Design review of the part built by this model. Coordinates are the model's own, in mm. Give positions to 0.01 mm unless a question says otherwise; leave off trailing zeros. Order: outer loops, then holes, each group sorted by start corner. A loop starts at its lowest first (then second) coordinate and runs counter-clockwise, first axis right, second up. Notation, with made-up numbers: (89.5, -11) -> (100.5, -11) arc R15 ccw to (100.5, 12) -> close; hole circle Ø9 at (88, -19.75). An arc over 180 degrees is marked (long way). One line per item, written item: value.
from build123d import *

# Parameters (mm, degrees)
SZKIC1_R                        = 6
SZKIC1_R_2                      = 1.6
SZKIC1_R_3                      = 2.15
DODANIE_WYCI_GNI_CIE1_DEPTH     = 5
ZAOKR_GLENIE1_R                 = 20
SFAZOWANIE1_SIZE                = 1
SZKIC2_R                        = 3.05
WYTNIJ_WYCI_GNI_CIE1_DEPTH      = 1.0000001
WYTNIJ_WYCI_GNI_CIE1_DEPTH_BACK = 6.0000001
SZKIC3_R                        = 2.25
WYTNIJ_WYCI_GNI_CIE2_DEPTH      = 1.0000001
WYTNIJ_WYCI_GNI_CIE2_DEPTH_BACK = 6.0000001
SZKIC4_R                        = 5
WYTNIJ_WYCI_GNI_CIE3_DEPTH      = 16
SZKIC5_R                        = 6
WYTNIJ_WYCI_GNI_CIE4_DEPTH      = 10
SZKIC6_R                        = 1.575
WYTNIJ_WYCI_GNI_CIE5_DEPTH      = 10
SFAZOWANIE2_SIZE                = 1


with BuildPart() as part:
    # Szkic1 → Dodanie-wyci_gni_cie1 (new body)
    with BuildSketch(Plane.XY):
        with BuildLine():
            ThreePointArc((117.467013895, 64.47868366), (93.021164267, 71.454105589), (67.678172045, 73.451308732))
            Line((67.678172045, 73.451308732), (-67.678172045, 73.451308732))
            ThreePointArc((-67.678172045, 73.451308732), (-93.021164267, 71.454105589), (-117.467013895, 64.47868366))
            ThreePointArc((-117.467013895, 64.47868366), (-133.996600631, 0.95447329), (-118.373625878, -62.798763495))
            ThreePointArc((-118.373625878, -62.798763495), (-114.037971639, -67.832241049), (-107.953613934, -70.499521549))
            ThreePointArc((-107.953613934, -70.499521549), (0, -80.778253493), (107.953613934, -70.499521549))
            ThreePointArc((107.953613934, -70.499521549), (114.037971639, -67.832241049), (118.373625878, -62.798763495))
            ThreePointArc((118.373625878, -62.798763495), (133.996600631, 0.95447329), (117.467013895, 64.47868366))
        make_face()
        with Locations((-79.843156229, -62.51471301)):
            Circle(SZKIC1_R, mode=Mode.SUBTRACT)
        with Locations((-60, -65.014543178)):
            Circle(SZKIC1_R, mode=Mode.SUBTRACT)
        with BuildLine():
            Line((-93.639920436, -10.215979742), (-85.426816489, -11.936656557))
            ThreePointArc((-85.426816489, -11.936656557), (-69.154538898, -19.133220925), (-57.227836692, -32.336679986))
            add(Edge.make_bspline(
                [(-72.285057891, -50.981377576), (-64.366611345, -52.03697099), (-50.388689008, -44.15086566), (-57.227836692, -32.336679986)],
                knots=[0, 0, 0, 0, 1, 1, 1, 1], degree=3))
            ThreePointArc((-72.285057891, -50.981377576), (-83.943779984, -49.299228552), (-95.563579221, -47.366434753))
            ThreePointArc((-95.563579221, -47.366434753), (-101.119264644, -44.79470717), (-104.683334782, -39.817074466))
            ThreePointArc((-104.683334782, -39.817074466), (-107.042286981, -32.953737236), (-108.951787413, -25.952033051))
            ThreePointArc((-108.951787413, -25.952033051), (-105.622705702, -13.873790687), (-93.639920436, -10.215979742))
        make_face(mode=Mode.SUBTRACT)
        with Locations((60, -65.014543178)):
            Circle(SZKIC1_R, mode=Mode.SUBTRACT)
        with Locations((79.843156229, -62.51471301)):
            Circle(SZKIC1_R, mode=Mode.SUBTRACT)
        with BuildLine():
            ThreePointArc((57.227836692, -32.336679986), (69.154538898, -19.133220925), (85.426816489, -11.936656557))
            Line((85.426816489, -11.936656557), (93.639920436, -10.215979742))
            ThreePointArc((93.639920436, -10.215979742), (105.622705702, -13.873790687), (108.951787413, -25.952033051))
            ThreePointArc((108.951787413, -25.952033051), (107.042286981, -32.953737236), (104.683334782, -39.817074466))
            ThreePointArc((104.683334782, -39.817074466), (101.119264644, -44.79470717), (95.563579221, -47.366434753))
            ThreePointArc((95.563579221, -47.366434753), (83.943779984, -49.299228552), (72.285057891, -50.981377576))
            add(Edge.make_bspline(
                [(72.285057891, -50.981377576), (64.366611345, -52.03697099), (50.388689008, -44.15086566), (57.227836692, -32.336679986)],
                knots=[0, 0, 0, 0, 1, 1, 1, 1], degree=3))
        make_face(mode=Mode.SUBTRACT)
        with BuildLine():
            Line((-74.826032056, 11.014530402), (-96.655711946, 16.415211274))
            ThreePointArc((-96.655711946, 16.415211274), (-105.521825108, 23.188783802), (-106.621107385, 34.291973698))
            ThreePointArc((-106.621107385, 34.291973698), (-104.340687454, 40.706522101), (-101.674756414, 46.970670723))
            ThreePointArc((-101.674756414, 46.970670723), (-91.74794023, 55.218917354), (-79.089039168, 52.703469899))
            ThreePointArc((-79.089039168, 52.703469899), (-75.870232147, 50.506568408), (-72.478506287, 48.587378348))
            ThreePointArc((-72.478506287, 48.587378348), (-63.066485572, 41.379596603), (-56.80899086, 31.310733134))
            add(Edge.make_bspline(
                [(-58.521368144, 15.244283258), (-55.163116948, 18.373947188), (-54.683502949, 25.918210288), (-56.80899086, 31.310733134)],
                knots=[0, 0, 0, 0, 1, 1, 1, 1], degree=3))
            ThreePointArc((-58.521368144, 15.244283258), (-66.137786774, 11.063591883), (-74.826032056, 11.014530402))
        make_face(mode=Mode.SUBTRACT)
        with BuildLine():
            Line((96.655711946, 16.415211274), (74.826032056, 11.014530402))
            ThreePointArc((74.826032056, 11.014530402), (66.137786774, 11.063591883), (58.521368144, 15.244283258))
            add(Edge.make_bspline(
                [(58.521368144, 15.244283258), (55.163116948, 18.373947188), (54.683502949, 25.918210288), (56.80899086, 31.310733134)],
                knots=[0, 0, 0, 0, 1, 1, 1, 1], degree=3))
            ThreePointArc((56.80899086, 31.310733134), (63.066485572, 41.379596603), (72.478506287, 48.587378348))
            ThreePointArc((72.478506287, 48.587378348), (75.870232147, 50.506568408), (79.089039168, 52.703469899))
            ThreePointArc((79.089039168, 52.703469899), (91.74794023, 55.218917354), (101.674756414, 46.970670723))
            ThreePointArc((101.674756414, 46.970670723), (104.340687454, 40.706522101), (106.621107385, 34.291973698))
            ThreePointArc((106.621107385, 34.291973698), (105.521825108, 23.188783802), (96.655711946, 16.415211274))
        make_face(mode=Mode.SUBTRACT)
        with Locations((-29, 59)):
            Circle(SZKIC1_R_2, mode=Mode.SUBTRACT)
        with Locations((29, 59)):
            Circle(SZKIC1_R_2, mode=Mode.SUBTRACT)
        with Locations((39, 45.817716041)):
            Circle(SZKIC1_R_2, mode=Mode.SUBTRACT)
        with Locations((-39, 45.817716041)):
            Circle(SZKIC1_R_2, mode=Mode.SUBTRACT)
        with Locations((-49, 24)):
            Circle(SZKIC1_R_3, mode=Mode.SUBTRACT)
        with Locations((49, 24)):
            Circle(SZKIC1_R_3, mode=Mode.SUBTRACT)
        with Locations((-49, -34)):
            Circle(SZKIC1_R_3, mode=Mode.SUBTRACT)
        with Locations((49, -34)):
            Circle(SZKIC1_R_3, mode=Mode.SUBTRACT)
        with Locations((48.501518409, -72.659085912)):
            Circle(SZKIC1_R_2, mode=Mode.SUBTRACT)
        with Locations((-48.501518409, -72.659085912)):
            Circle(SZKIC1_R_2, mode=Mode.SUBTRACT)
    extrude(amount=DODANIE_WYCI_GNI_CIE1_DEPTH)

    # Zaokr_glenie1
    zaokr_glenie1_edges = [part.edges().sort_by_distance(p)[0] for p in [
        (117.467013895, 64.47868366, 2.5),
        (-117.467013895, 64.47868366, 2.5),
    ]]
    fillet(zaokr_glenie1_edges, radius=ZAOKR_GLENIE1_R)

    # Sfazowanie1
    sfazowanie1_edges = [part.edges().sort_by_distance(p)[0] for p in [
        (-50.101518409, -72.659085912, 0),
        (46.901518409, -72.659085912, 0),
        (46.85, -34, 0),
        (37.4, 45.817716041, 0),
        (-40.6, 45.817716041, 0),
        (-51.15, 24, 0),
        (46.85, 24, 0),
        (-51.15, -34, 0),
        (-30.6, 59, 0),
        (27.4, 59, 0),
    ]]
    chamfer(sfazowanie1_edges, length=SFAZOWANIE1_SIZE)

    # Szkic2 → Wytnij-wyci_gni_cie1 (cut, two sides)
    with BuildSketch(Plane.XY.offset(5)) as wytnij_wyci_gni_cie1_sk:
        with Locations((0.003475223, -29.063691268)):
            Circle(SZKIC2_R)
        with Locations((22.00052048, 9.036308732)):
            Circle(SZKIC2_R)
        with Locations((-21.993570033, 9.036308732)):
            Circle(SZKIC2_R)
    extrude(amount=WYTNIJ_WYCI_GNI_CIE1_DEPTH, mode=Mode.SUBTRACT)
    extrude(wytnij_wyci_gni_cie1_sk.sketch, amount=-WYTNIJ_WYCI_GNI_CIE1_DEPTH_BACK, mode=Mode.SUBTRACT)

    # Szkic3 → Wytnij-wyci_gni_cie2 (cut, two sides)
    with BuildSketch(Plane(origin=(0, 0, 0), x_dir=(-1, 0, 0), z_dir=(0, 0, -1))) as wytnij_wyci_gni_cie2_sk:
        with Locations((114.588433544, 44.704484093)):
            Circle(SZKIC3_R)
        with Locations((119.652409391, -28.500893439)):
            Circle(SZKIC3_R)
        with Locations((-119.652409391, -28.500893439)):
            Circle(SZKIC3_R)
        with Locations((-114.588433544, 44.704484093)):
            Circle(SZKIC3_R)
    extrude(amount=WYTNIJ_WYCI_GNI_CIE2_DEPTH, mode=Mode.SUBTRACT)
    extrude(wytnij_wyci_gni_cie2_sk.sketch, amount=-WYTNIJ_WYCI_GNI_CIE2_DEPTH_BACK, mode=Mode.SUBTRACT)

    # Szkic4 → Wytnij-wyci_gni_cie3 (cut)
    with BuildSketch(Plane(origin=(0, 0, 0), x_dir=(-1, 0, 0), z_dir=(0, 0, -1))):
        with Locations((0.11301634, 43.451308732)):
            Circle(SZKIC4_R)
        with Locations((-27.88698366, 34.451308732)):
            Circle(SZKIC4_R)
        with Locations((28.11301634, 34.451308732)):
            Circle(SZKIC4_R)
    extrude(amount=-WYTNIJ_WYCI_GNI_CIE3_DEPTH, mode=Mode.SUBTRACT)

    # Szkic5 → Wytnij-wyci_gni_cie4 (cut)
    with BuildSketch(Plane(origin=(0, 0, 0), x_dir=(-1, 0, 0), z_dir=(0, 0, -1))):
        with Locations((44, -20)):
            Circle(SZKIC5_R)
        with Locations((-44, -20)):
            Circle(SZKIC5_R)
    extrude(amount=-WYTNIJ_WYCI_GNI_CIE4_DEPTH, mode=Mode.SUBTRACT)

    # Szkic6 → Wytnij-wyci_gni_cie5 (cut)
    with BuildSketch(Plane(origin=(0, 0, 0), x_dir=(-1, 0, 0), z_dir=(0, 0, -1))):
        with Locations((105.78946688, -56.662469542)):
            Circle(SZKIC6_R)
        with Locations((-105.78946688, -56.662469542)):
            Circle(SZKIC6_R)
    extrude(amount=-WYTNIJ_WYCI_GNI_CIE5_DEPTH, mode=Mode.SUBTRACT)

    # Sfazowanie2
    sfazowanie2_edges = [part.edges().sort_by_distance(p)[0] for p in [
        (-104.21446688, -56.662469542, 0),
        (107.36446688, -56.662469542, 0),
    ]]
    chamfer(sfazowanie2_edges, length=SFAZOWANIE2_SIZE)


solid = part.part
Item 1: Clearance check with a flat-ended pin moving along its axis: P1, Ø11, axis at x = 44, y = -20, coming from the -Z side. State where the tip first meets the part, or that it passes through.
Returned:
P1: through
Item 2: Add section A-A on y = -20. Give the boundary of the cut face in (x, z), plus the area to 3 significant figures.
Returned:
outline: (-132.5, 0) -> (-108.97, 0) -> (-108.97, 5) -> (-132.5, 5) -> close; (-68, 0) -> (-50, 0) -> (-50, 5) -> (-68, 5) -> close; (-38, 0) -> (38, 0) -> (38, 5) -> (-38, 5) -> close; (50, 0) -> (68, 0) -> (68, 5) -> (50, 5) -> close; (108.97, 0) -> (132.5, 0) -> (132.5, 5) -> (108.97, 5) -> close
area: 795 mm²
Item 3: To check wall thickness, follow line 1 along Y through (x, z) = (-67, 0.2); line 2 along Y through (x, z) = (-68.5, 4.05); line 3 along X through (y, z) = (-67, 1.35). State the ranges of each line that lie inside material, in increasing order. Write a range as from..to.
Returned:
line 1: -76.84..-50.58, -20.8..10.86, 45.06..73.45
line 2: -76.66..-50.89, -19.62..10.62, 46.18..73.47
line 3: -115.07..-83.83, -75.86..-65.66, -54.34..54.34, 65.66..75.86, 83.83..115.07
Item 4: Draft analysis for pull direction X (two halves, no side actions). For faces 1 (the cylindrical face through (-0.66, -32.04, 2.54)), 2 (the cylindrical face through (-1.52, -80.776, 2.465)), 3 (the cylindrical face through (-133.977, -2.472, 2.465)), state which applies: pulls with the +X half, pulls with the -X half, needs draft (parallel to the pull), parting line crosses it, or undercut.
Returned:
face 1: undercut
face 2: parting line crosses it
face 3: pulls with the -X half
Item 5: Add section B-B on x = -91. Give the boundary of the cut face in (y, z).
Returned:
outline: (-73.49, 0) -> (-48.16, 0) -> (-48.16, 5) -> (-73.49, 5) -> close; (-10.77, 0) -> (15.02, 0) -> (15.02, 5) -> (-10.77, 5) -> close; (55.39, 0) -> (71.8, 0) -> (71.8, 5) -> (55.39, 5) -> close
